Autodesk Inventor part; units mm, degrees
ref_plane "YZ Plane" through (0, 0, 0) normal (1, 0, 0) x (0, 1, 0)
ref_plane "XZ Plane" through (0, 0, 0) normal (0, 1, 0) x (-1, 0, 0)
ref_plane "XY Plane" through (0, 0, 0) normal (0, 0, 1) x (1, 0, 0)
sketch "Esboço1" plane through (0, 0, 0) normal (0, 0, 1) x (1, 0, 0)
  circle A0 centre (0, 0) radius 7.5
  circle A1 centre (0, 0) radius 6
  dimension "d0" = 15
  dimension "d1" = 12
extrude "Extrusão1" add sketch "Esboço1" along normal blind 12
sketch "Esboço2" plane through (0, 0, 0) normal (0, 0, -1) x (-1, 0, 0)
  circle A0 centre (0, 0) radius 6
extrude "Extrusão2" add sketch "Esboço2" against normal blind 11
fillet "Arredondamento1" radius 0.3 2 edges at (-7.5, 0, 12) (-6, 0, 11)
properties part number "Caixa"
Design review of the part built by this model. Coordinates are the model's own, in mm. A direction names the side the tool comes from. Coordinates: 2 decimals unless noted, no trailing zeros. Order: outer loops, then holes, each group sorted by start corner. A loop starts at its lowest first (then second) coordinate and runs counter-clockwise, first axis right, second up. Notation, with made-up numbers: M 53,-27.75 L 76,-27.75 A24 cw 76,-15.75 Z; hole C 7.25,56.5 d8. An arc over 180 degrees is marked long. Use a Markdown table: item, result.
(1) Draft analysis for pull direction Y (two halves, no side actions). For faces 1 (the cylindrical face through (-7.493, -0.33, 5.768)), 2 (the cylindrical face through (-5.994, -0.264, 11.645)), 3 (the flat face through (-2, 6, 12)), state which applies: released by +Y, released by -Y, zero draft, split by the parting line, or undercut.
Worked answers:
| item | result |
|---|---|
| face 1 | split by the parting line |
| face 2 | undercut |
| face 3 | zero draft |
(2) For P1, Ø4, axis at y = -2.5, z = 9, coming from the -X side; P2, Ø1.5, axis at x = -2, y = -0.5, coming from the +Z side; P3, Ø1, axis at x = -3, z = 5, coming from the +Y side, all flat-tipped, find the tip position at first contact; note any pin that passes through.
Worked answers:
| item | result |
|---|---|
| P1 | stops at x = -7.48 |
| P2 | stops at z = 11 |
| P3 | stops at y = 7.07 |
(3) Add section C-C (z = 1.5). Give the boundary of the cut face in (x, y), then the cut area to 3 significant figures.
Worked answers:
| item | result |
|---|---|
| outline | C 0,0 d15 |
| area | 177 mm2 |
(4) Add section A-A (y = 0). Give the boundary of the cut face in (x, z).
Worked answers:
| item | result |
|---|---|
| outline | M -7.5,0 L 7.5,0 L 7.5,11.7 A0.3 ccw 7.2,12 L 6,12 L 6,11.3 A0.3 cw 5.7,11 L -5.7,11 A0.3 cw -6,11.3 L -6,12 L -7.2,12 A0.3 ccw -7.5,11.7 Z |
(5) Wall thickness on probe 1 along Y at (x, z) = (0, 11.6); probe 2 along X at (y, z) = (0.25, 6.5); probe 3 along Z at (x, y) = (2.5, -1.25): over which ranges is each line inside the solid? List them lowest first.
Worked answers:
| item | result |
|---|---|
| probe 1 | y = -7.5 to -6, 6 to 7.5 |
| probe 2 | x = -7.5 to 7.5 |
| probe 3 | z = 0 to 11 |
(6) For faces 4 (the flat face through (0, 0, 11)), 5 (the flat face through (0, 0, 0)), list the 3-axis set-ups (+Z, -Z, +X, -X, +Y, -Y) from which the entire face can be reached by the end or side of a thin tool; tool diameter is ignored.
Worked answers:
| item | result |
|---|---|
| face 4 | +Z |
| face 5 | -Z, +X, -X, +Y, -Y |
